Verification items for this drawing (mm, ordinates from the low corner). A direction names the side the tool comes from. Round coordinates to 2 decimals unless told otherwise and drop trailing zeros. Write each loop counter-clockwise with the first axis right and the second up, starting at its lowest first coordinate (ties: lowest second). Pieces come first, ordered by that corner, then holes. Notation, with made-up numbers: (-9, 35) -> (-4, 35) arc R27 ccw to (-4, 54) -> close; hole circle Ø4 at (-30, 7.5). An arc over 180 degrees is marked (long way). One line per item, written item: value.
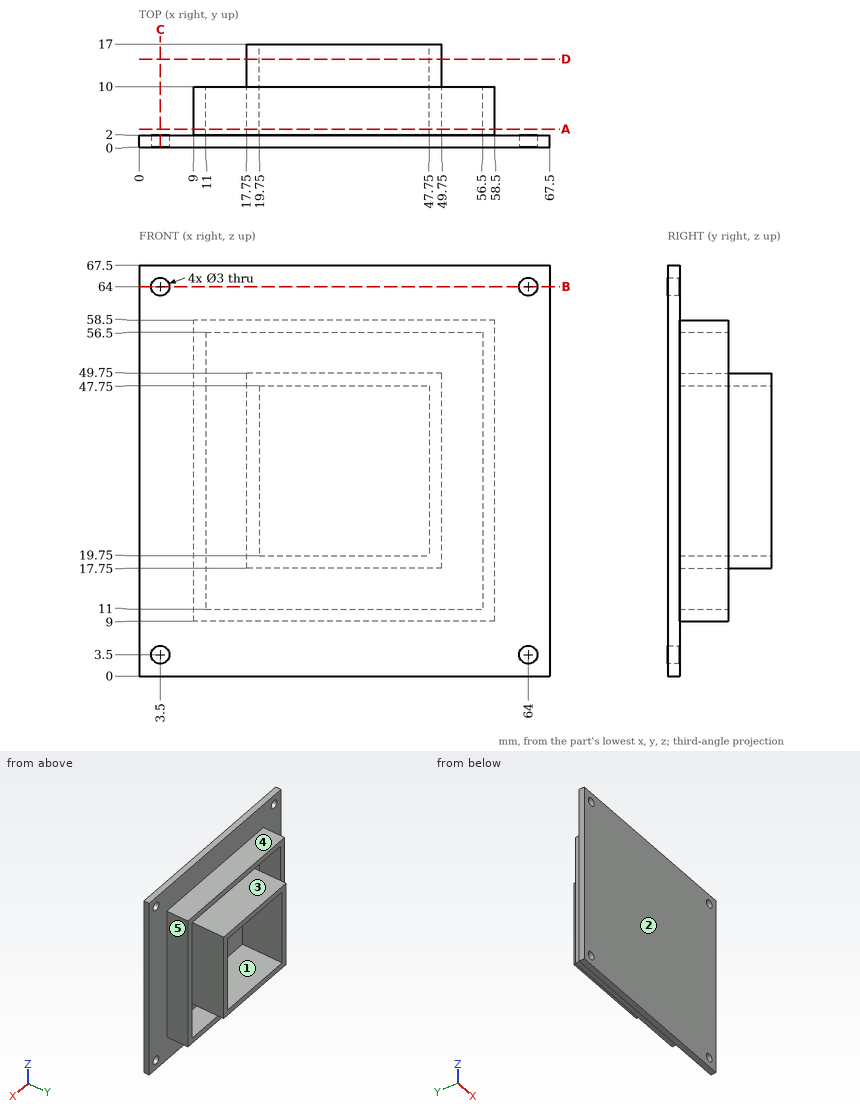
Item 1: Sectioned sample at C-C (x = 3.5). Enter the section's corners in (y, z).
Result set:
outline: (0, 0) -> (2, 0) -> (2, 2) -> (0, 2) -> close; (0, 5) -> (2, 5) -> (2, 62.5) -> (0, 62.5) -> close; (0, 65.5) -> (2, 65.5) -> (2, 67.5) -> (0, 67.5) -> close
Item 2: Tool access check on the marked faces 1 and 2. Record the directions out of +Z, -Z, +X, -X, +Y, -Y that give a thin tool (end or side, any length) a straight path to the whole face; none if there is none.
Result set:
face 1: +Y
face 2: +Z, -Z, +X, -X, -Y
Item 3: Sectioned sample at A-A (y = 3). Enter the section's corners in (x, z).
Result set:
outline: (9, 9) -> (58.5, 9) -> (58.5, 58.5) -> (9, 58.5) -> close; (17.75, 17.75) -> (49.75, 17.75) -> (49.75, 49.75) -> (17.75, 49.75) -> close; hole (11, 11) -> (56.5, 11) -> (56.5, 56.5) -> (11, 56.5) -> close; hole (19.75, 19.75) -> (47.75, 19.75) -> (47.75, 47.75) -> (19.75, 47.75) -> close
Item 4: Release check for a two-part mould opening along X. For the marked faces 3, 4 and 5 record: pulls with the +X half, pulls with the -X half, needs draft (parallel to the pull), parting line crosses it, or undercut.
Result set:
face 3: undercut
face 4: needs draft
face 5: pulls with the +X half
Item 5: Sectioned sample at B-B (z = 64). Enter the section's corners in (x, y), then the cut area to 3 significant figures.
Result set:
outline: (0, 0) -> (2, 0) -> (2, 2) -> (0, 2) -> close; (5, 0) -> (62.5, 0) -> (62.5, 2) -> (5, 2) -> close; (65.5, 0) -> (67.5, 0) -> (67.5, 2) -> (65.5, 2) -> close
area: 123 mm^2
Item 6: Depth check by flat-ended pin: pin 1 (5 mm diameter, centred on x = 59.5, z = 9.5, fed in from -Y); pin 2 (4.5 mm diameter, centred on x = 36, y = 6, fed in from -Z); pin 3 (7.5 mm diameter, centred on y = 10, z = 33, fed in from +X); pin 4 (4 mm diameter, centred on x = 3.5, z = 3.5, fed in from +Y). Enter the tip coordinate at first touch or a pass-through.
Result set:
pin 1: y = 0
pin 2: z = 9
pin 3: x = 58.5
pin 4: y = 2
Item 7: Material ranges on line 1 along Z through (x, y) = (32, 2.5); line 2 along X through (y, z) = (1.35, 3.5), recorded low to high.
Result set:
line 1: 9 to 11, 17.75 to 19.75, 47.75 to 49.75, 56.5 to 58.5
line 2: 0 to 2, 5 to 62.5, 65.5 to 67.5
Item 8: Sectioned sample at D-D (y = 14.5). Enter the section's corners in (x, z), then the cut area to 3 significant figures.
Result set:
outline: (17.75, 17.75) -> (49.75, 17.75) -> (49.75, 49.75) -> (17.75, 49.75) -> close; hole (19.75, 19.75) -> (47.75, 19.75) -> (47.75, 47.75) -> (19.75, 47.75) -> close
area: 240 mm^2
